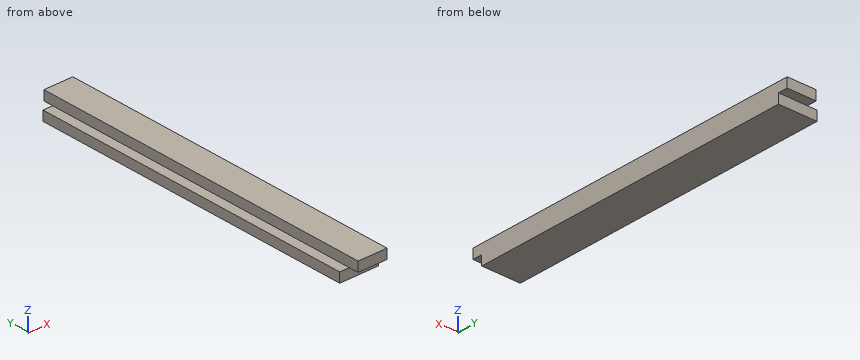
from build123d import *

# Parameters (mm, degrees)
SKETCH1_W           = 40
SKETCH1_H           = 360
BOSS_EXTRUDE1_DEPTH = 20
SKETCH2_W           = 10
SKETCH2_H           = 360
CUT_EXTRUDE1_DEPTH  = 10
SKETCH3_W           = 40
SKETCH3_H           = 10
CUT_EXTRUDE2_DEPTH  = 10


with BuildPart() as part:
    # Sketch1 → Boss-Extrude1 (new body)
    with BuildSketch(Plane.XY):
        Rectangle(SKETCH1_W, SKETCH1_H)
    extrude(amount=BOSS_EXTRUDE1_DEPTH)

    # Sketch2 → Cut-Extrude1 (cut)
    with BuildSketch(Plane.XY.offset(20)):
        with Locations((-15, 0)):
            Rectangle(SKETCH2_W, SKETCH2_H)
    extrude(amount=-CUT_EXTRUDE1_DEPTH, mode=Mode.SUBTRACT)

    # Sketch3 → Cut-Extrude2 (cut)
    with BuildSketch(Plane(origin=(0, 0, 0), x_dir=(-1, 0, 0), z_dir=(0, 0, -1))):
        with Locations((0, 175)):
            Rectangle(SKETCH3_W, SKETCH3_H)
        with Locations((0, -175)):
            Rectangle(SKETCH3_W, SKETCH3_H)
    extrude(amount=-CUT_EXTRUDE2_DEPTH, mode=Mode.SUBTRACT)


solid = part.part
The listing builds one solid part. Answer for the finished solid, in the listing's coordinates (mm). Coordinates: 2 decimals unless noted, no trailing zeros. Order: outer loops, then holes, each group sorted by start corner. A loop starts at its lowest first (then second) coordinate and runs counter-clockwise, first axis right, second up. Notation, with made-up numbers: M -16.75,72.5 L 4.25,72.5 A30 cw 4.25,98.5 Z; hole C 77,25 d9. An arc over 180 degrees is marked long. Use CSV: the item, a comma, the result in double quotes.
Q1. Given pin 1 Ø3 at (y, z) = (53.5, 15.5) entering from -X; pin 2 Ø8 at (x, y) = (1, -176) entering from -Z; pin 3 Ø5 at (x, y) = (-13.5, 45.5) entering from +Z, each flat-ended and moving along its own axis, determine where each tip first touches the part or whether it passes through.
Here are the results:
pin 1,"x = -10"
pin 2,"z = 10"
pin 3,"z = 10"
Q2. Section A-A (x = 16) is taken. Determine the outline of the cut face in (y, z).
Here are the results:
outline,"M -180,10 L -170,10 L -170,0 L 170,0 L 170,10 L 180,10 L 180,20 L -180,20 Z"
Q3. Straight lines are drawn through the part: L1, parallel to X at y = 70, z = 12.25; L2, parallel to Y at x = -17, z = 9.5; L3, parallel to Z at x = -17.5, y = 145. For each, find the intervals that lie inside material, in ascending order.
Here are the results:
L1,"-10 to 20"
L2,"-170 to 170"
L3,"0 to 10"
Q4. Section B-B (z = 7) is taken. Determine the outline of the cut face in (x, y), then the cut area to 3 significant figures.
Here are the results:
outline,"M -20,-170 L 20,-170 L 20,170 L -20,170 Z"
area,"13,600 mm2"
Q5. Section C-C (y = 144) is taken. Determine the outline of the cut face in (x, z).
Here are the results:
outline,"M -20,0 L 20,0 L 20,20 L -10,20 L -10,10 L -20,10 Z"
